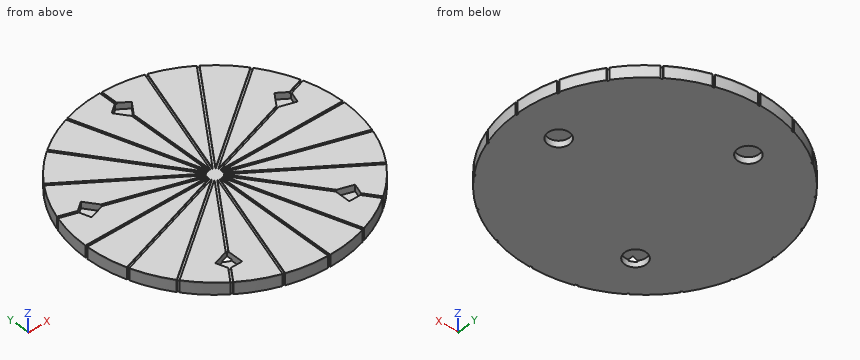
from build123d import *

# Parameters (mm, degrees)
F0_R            = 60
F1_DEPTH        = 5
F3_DEPTH        = 0.5
F4_W            = 5
F4_H            = 1
F5_DEPTH        = 5.501
F5_COPIES_COUNT = 20
F8_DEPTH        = 3
F9_R            = 5
F10_DEPTH       = 3


# Not quite as in the source:
# - a pattern or mirror of a feature is missing from the dataset's text; its kind, count and spacing are read off the source's solid


with BuildPart() as f1:
    # F0 (on Top) → F1 (new body)
    with BuildSketch(Plane.XY):
        Circle(F0_R)
    extrude(amount=F1_DEPTH)

    # F2 (on face) → F3 (join)
    with BuildSketch(Plane.XY.offset(5)):
        with BuildLine():
            ThreePointArc((59.9979166305, 0.5), (59.2613004357, 9.3860679024), (57.2159180728, 18.0648476078))
            Line((57.2159180728, 18.0648476078), (3.1568757573, 0.5))
            Line((3.1568757573, 0.5), (59.9979166305, 0.5))
        make_face()
        with BuildLine():
            ThreePointArc((56.9069010784, 19.0159041241), (53.4603914513, 27.2394299844), (48.8332268073, 34.8613820665))
            Line((48.8332268073, 34.8613820665), (2.847858763, 1.4510565163))
            Line((2.847858763, 1.4510565163), (56.9069010784, 19.0159041241))
        make_face()
        with BuildLine():
            ThreePointArc((48.245441555, 35.6703990609), (42.4264068712, 42.4264068712), (35.6703990609, 48.245441555))
            Line((35.6703990609, 48.245441555), (2.2600735107, 2.2600735107))
            Line((2.2600735107, 2.2600735107), (48.245441555, 35.6703990609))
        make_face()
        with BuildLine():
            ThreePointArc((34.8613820665, 48.8332268073), (27.2394299844, 53.4603914513), (19.0159041241, 56.9069010784))
            Line((19.0159041241, 56.9069010784), (1.4510565163, 2.847858763))
            Line((1.4510565163, 2.847858763), (34.8613820665, 48.8332268073))
        make_face()
        with BuildLine():
            ThreePointArc((18.0648476078, 57.2159180728), (9.3860679024, 59.2613004357), (0.5, 59.9979166305))
            Line((0.5, 59.9979166305), (0.5, 3.1568757573))
            Line((0.5, 3.1568757573), (18.0648476078, 57.2159180728))
        make_face()
        with BuildLine():
            ThreePointArc((-0.5, 59.9979166305), (-9.3860679024, 59.2613004357), (-18.0648476078, 57.2159180728))
            Line((-18.0648476078, 57.2159180728), (-0.5, 3.1568757573))
            Line((-0.5, 3.1568757573), (-0.5, 59.9979166305))
        make_face()
        with BuildLine():
            ThreePointArc((-19.0159041241, 56.9069010784), (-27.2394299844, 53.4603914513), (-34.8613820665, 48.8332268073))
            Line((-34.8613820665, 48.8332268073), (-1.4510565163, 2.847858763))
            Line((-1.4510565163, 2.847858763), (-19.0159041241, 56.9069010784))
        make_face()
        with BuildLine():
            ThreePointArc((-35.6703990609, 48.245441555), (-42.4264068712, 42.4264068712), (-48.245441555, 35.6703990609))
            Line((-48.245441555, 35.6703990609), (-2.2600735107, 2.2600735107))
            Line((-2.2600735107, 2.2600735107), (-35.6703990609, 48.245441555))
        make_face()
        with BuildLine():
            ThreePointArc((-48.8332268073, 34.8613820665), (-53.4603914513, 27.2394299844), (-56.9069010784, 19.0159041241))
            Line((-56.9069010784, 19.0159041241), (-2.847858763, 1.4510565163))
            Line((-2.847858763, 1.4510565163), (-48.8332268073, 34.8613820665))
        make_face()
        with BuildLine():
            ThreePointArc((-57.2159180728, 18.0648476078), (-59.2613004357, 9.3860679024), (-59.9979166305, 0.5))
            Line((-59.9979166305, 0.5), (-3.1568757573, 0.5))
            Line((-3.1568757573, 0.5), (-57.2159180728, 18.0648476078))
        make_face()
        with BuildLine():
            Line((-3.1568757573, -0.5), (-59.9979166305, -0.5))
            ThreePointArc((-59.9979166305, -0.5), (-59.2613004357, -9.3860679024), (-57.2159180728, -18.0648476078))
            Line((-57.2159180728, -18.0648476078), (-3.1568757573, -0.5))
        make_face()
        with BuildLine():
            Line((-2.847858763, -1.4510565163), (-56.9069010784, -19.0159041241))
            ThreePointArc((-56.9069010784, -19.0159041241), (-53.4603914513, -27.2394299844), (-48.8332268073, -34.8613820665))
            Line((-48.8332268073, -34.8613820665), (-2.847858763, -1.4510565163))
        make_face()
        with BuildLine():
            Line((-2.2600735107, -2.2600735107), (-48.245441555, -35.6703990609))
            ThreePointArc((-48.245441555, -35.6703990609), (-42.4264068712, -42.4264068712), (-35.6703990609, -48.245441555))
            Line((-35.6703990609, -48.245441555), (-2.2600735107, -2.2600735107))
        make_face()
        with BuildLine():
            Line((-1.4510565163, -2.847858763), (-34.8613820665, -48.8332268073))
            ThreePointArc((-34.8613820665, -48.8332268073), (-27.2394299844, -53.4603914513), (-19.0159041241, -56.9069010784))
            Line((-19.0159041241, -56.9069010784), (-1.4510565163, -2.847858763))
        make_face()
        with BuildLine():
            Line((-0.5, -3.1568757573), (-18.0648476078, -57.2159180728))
            ThreePointArc((-18.0648476078, -57.2159180728), (-9.3860679024, -59.2613004357), (-0.5, -59.9979166305))
            Line((-0.5, -59.9979166305), (-0.5, -3.1568757573))
        make_face()
        with BuildLine():
            Line((0.5, -3.1568757573), (0.5, -59.9979166305))
            ThreePointArc((0.5, -59.9979166305), (9.3860679024, -59.2613004357), (18.0648476078, -57.2159180728))
            Line((18.0648476078, -57.2159180728), (0.5, -3.1568757573))
        make_face()
        with BuildLine():
            Line((1.4510565163, -2.847858763), (19.0159041241, -56.9069010784))
            ThreePointArc((19.0159041241, -56.9069010784), (27.2394299844, -53.4603914513), (34.8613820665, -48.8332268073))
            Line((34.8613820665, -48.8332268073), (1.4510565163, -2.847858763))
        make_face()
        with BuildLine():
            Line((2.2600735107, -2.2600735107), (35.6703990609, -48.245441555))
            ThreePointArc((35.6703990609, -48.245441555), (42.4264068712, -42.4264068712), (48.245441555, -35.6703990609))
            Line((48.245441555, -35.6703990609), (2.2600735107, -2.2600735107))
        make_face()
        with BuildLine():
            Line((2.847858763, -1.4510565163), (48.8332268073, -34.8613820665))
            ThreePointArc((48.8332268073, -34.8613820665), (53.4603914513, -27.2394299844), (56.9069010784, -19.0159041241))
            Line((56.9069010784, -19.0159041241), (2.847858763, -1.4510565163))
        make_face()
        with BuildLine():
            Line((3.1568757573, -0.5), (57.2159180728, -18.0648476078))
            ThreePointArc((57.2159180728, -18.0648476078), (59.2613004357, -9.3860679024), (59.9979166305, -0.5))
            Line((59.9979166305, -0.5), (3.1568757573, -0.5))
        make_face()
    extrude(amount=F3_DEPTH)

    # F4 (on face) → F5 (cut, through all)
    with BuildSketch(Plane.XY.offset(5.5)):
        with Locations((-61.9979166305, 0)):
            Rectangle(F4_W, F4_H)
    f5 = extrude(amount=-F5_DEPTH, mode=Mode.SUBTRACT)

    # F5_copies: F5 ×20 about axis
    f5_copies_axis = Axis((0, 0, 0), (0, 0, 1))
    for i in range(1, F5_COPIES_COUNT):
        add(f5.rotate(f5_copies_axis, i * 360 / F5_COPIES_COUNT), mode=Mode.SUBTRACT)

    # F7 (on face) → F8 (cut)
    with BuildSketch(Plane.XY.offset(5.5)):
        Polygon((-4.7022820183, 49.0046763726), (0, 42.5325404176), (4.7022820183, 49.0046763726), (0, 52.4210842376), align=None)
        Polygon((-48.0593018491, 10.671141848), (-40.4508497187, 13.143277803), (-40.9508497187, 13.8314687632), (-49.3554137554, 16.562277157), (-49.8554137554, 16.199005893), align=None)
        Polygon((-49.3554137554, 16.562277157), (-40.9508497187, 13.8314687632), (-45.1531317371, 19.615413758), align=None)
        Polygon((45.1531317371, 19.615413758), (40.4508497187, 13.143277803), (48.0593018491, 10.671141848), (49.8554137554, 16.199005893), align=None)
        Polygon((-25, -42.4095480118), (-25, -34.4095480118), (-32.6084521304, -36.8816839668), (-30.812340224, -42.4095480118), align=None)
        Polygon((32.6084521304, -36.8816839668), (25, -34.4095480118), (25, -42.4095480118), (30.812340224, -42.4095480118), align=None)
    extrude(amount=-F8_DEPTH, mode=Mode.SUBTRACT)

    # F9 (on face) → F10 (cut)
    with BuildSketch(Plane(origin=(0, 0, 0), x_dir=(1, 0, 0), z_dir=(0, 0, -1))):
        with Locations((-24.0012126607, 31.9990904686)):
            Circle(F9_R)
        with Locations((-15.5012126607, -36.87427838)):
            Circle(F9_R)
        with Locations((39.9987873393, 0.3114665041)):
            Circle(F9_R)
    extrude(amount=-F10_DEPTH, mode=Mode.SUBTRACT)


solid = f1.part
Geometry check sheet. Reference: the model listing, model coordinates, mm. Give positions to 0.01 mm unless a question says otherwise; leave off trailing zeros. Loops run counter-clockwise (first coordinate to the right, second up) from the corner with the lowest first, then second, coordinate; pieces in that order, holes last. Notation, with made-up numbers: M 8.5,-28 L 18.5,-28 A10 ccw 18.5,-9 Z; hole C 16,45.25 d2. An arc over 180 degrees is marked long. Answer as a JSON object with one key per item and string values. Group by question number.
Item 1: Sectioned sample at C-C on z = 3.9. Give the number of separate pieces and of enclosed holes in the cut face, plus the area to 3 significant figures.
Item 2: Gauge pin test, flat ends, axial feed: pin 1 (3 mm diameter, centred on x = 29.5, z = 0.5, fed in from -Y); pin 2 (3 mm diameter, centred on x = 37, z = 2.5, fed in from -Y); pin 3 (3 mm diameter, centred on x = 25.5, z = 3, fed in from +Y). Record the tip position at first contact, or that the pin passes through.
Item 3: Sectioned sample at A-A on x = -37.5. Record the boundary of the cut face in (y, z).
Item 4: Material ranges on L1, parallel to X at y = 14.5, z = 3.3; L2, parallel to X at y = -33, z = 1.8; L3, parallel to Y at x = 19.5, z = 1.45, recorded low to high.
Item 5: Sectioned sample at B-B on y = -39. Record the boundary of the cut face in (x, z), plus the area to 3 significant figures.
Findings below:
{
 "1": {"separate pieces": "1", "enclosed holes": "5", "area": "11,100 mm2"},
 "2": {"pin 1": "y = -53.07", "pin 2": "y = -48.25", "pin 3": "y = 54.99"},
 "3": {"outline": "M -46.84,0 L 46.84,0 L 46.84,5.5 L 27.86,5.5 L 27.86,5 L 26.63,5 L 26.63,5.5 L 12.71,5.5 L 12.71,5 L 11.66,5 L 11.66,5.5 L 0.5,5.5 L 0.5,5 L -0.5,5 L -0.5,5.5 L -11.66,5.5 L -11.66,5 L -12.71,5 L -12.71,5.5 L -26.63,5.5 L -26.63,5 L -27.86,5 L -27.86,5.5 L -46.84,5.5 Z"},
 "4": {"L1": "-58.22 to -49.3, -41.44 to 41.44, 49.3 to 58.22", "L2": "-50.11 to -28.9, -19.1 to 50.11", "L3": "-56.74 to 56.74"},
 "5": {"outline": "M -45.6,0 L 45.6,0 L 45.6,5.5 L 31.92,5.5 L 31.92,2.5 L 25,2.5 L 25,5.5 L 13.2,5.5 L 13.2,5 L 12.15,5 L 12.15,5.5 L 0.5,5.5 L 0.5,5 L -0.5,5 L -0.5,5.5 L -12.15,5.5 L -12.15,5 L -13.2,5 L -13.2,5.5 L -25,5.5 L -25,2.5 L -31.92,2.5 L -31.92,5.5 L -45.6,5.5 Z", "area": "458 mm2"}
}
